```python
from build123d import *

# Parameters (mm, degrees)
SKETCH_1_R      = 3.05
SKETCH_1_R_2    = 2.25
EXTRUDE_1_DEPTH = 7
SKETCH_2_R      = 5
SKETCH_2_R_2    = 2.25
EXTRUDE_2_DEPTH = 2
EXTRUDE_START   = -2
SKETCH_3_R      = 5
SKETCH_3_R_2    = 2.25
EXTRUDE_3_DEPTH = 2
CHAMFER_1_SIZE  = 1.5


with BuildPart() as part:
    # Эскиз1 → Вытянуть-Тонкостенный1 (new body)
    with BuildSketch(Plane(origin=(0, 0, 0), x_dir=(1, 0, 0), z_dir=(0, 1, 0))):
        Circle(SKETCH_1_R)
        Circle(SKETCH_1_R_2, mode=Mode.SUBTRACT)
    extrude(amount=EXTRUDE_1_DEPTH)

    # Эскиз2 → Вытянуть-Тонкостенный2 (add)
    with BuildSketch(Plane(origin=(0, 0, 0), x_dir=(1, 0, 0), z_dir=(0, 1, 0))):
        Circle(SKETCH_2_R)
        Circle(SKETCH_2_R_2, mode=Mode.SUBTRACT)
    extrude(amount=EXTRUDE_2_DEPTH)

    # Эскиз3 → Вытянуть-Тонкостенный3 (add)
    with BuildSketch(Plane(origin=(0, 7, 0), x_dir=(1, 0, 0), z_dir=(0, 1, 0)).offset(EXTRUDE_START)):
        Circle(SKETCH_3_R)
        Circle(SKETCH_3_R_2, mode=Mode.SUBTRACT)
    extrude(amount=EXTRUDE_3_DEPTH)

    # Фаска1
    chamfer_1_edges = [part.edges().sort_by_distance(p)[0] for p in [
        (-3.05, 2, 0),
        (-3.05, 5, 0),
    ]]
    chamfer(chamfer_1_edges, length=CHAMFER_1_SIZE - 0.0001)  # a hair under: the kernel refuses the full size


solid = part.part
```
Model file for the job. Use its own axes, mm. Give positions to 0.01 mm unless a question says otherwise; leave off trailing zeros. Write each loop counter-clockwise with the first axis right and the second up, starting at its lowest first coordinate (ties: lowest second). Pieces come first, ordered by that corner, then holes. Notation, with made-up numbers: M 61,8.5 L 88,8.5 A13 cw 88,24.5 Z; hole C 21.5,-29.75 d7. An arc over 180 degrees is marked long. Use a Markdown table: item, result.
1) Pin check, flat tips, straight feed: pin 1 (3.5 mm diameter, centred on x = 0, z = 0, fed in from -Y); pin 2 (2 mm diameter, centred on x = 2.5, y = 1.5, fed in from +Z). Stop position of each tip, or through.
Responses:
| item | result |
|---|---|
| pin 1 | passes through |
| pin 2 | stops at z = 4.77 |
2) Pull direction Z, two halves, no side cores. Call faces 1 (the cylindrical face through (-1.08, 5.99, 4.88)), 2 (the cylindrical face through (-0.29, 3.45, -2.23)), 3 (the flat face through (2.2, 7, 1)): +Z half, -Z half, draft (parallel to the pull), parting line (faces both ways), or undercut.
Responses:
| item | result |
|---|---|
| face 1 | parting line |
| face 2 | undercut |
| face 3 | draft |
3) Drill centre lines: line 1 (Y direction, x = 2.5, z = 4); line 2 (X direction, y = 5.75, z = 0). Where is each one in solid material? Low to high. Write a range as from..to.
Responses:
| item | result |
|---|---|
| line 1 | y = 0..2, 5..7 |
| line 2 | x = -5..-2.25, 2.25..5 |
4) Cut at C-C (y = 0.5). List the corners of the cut face in (x, z), and give its area (3 significant figures).
Responses:
| item | result |
|---|---|
| outline | C 0,0 d10; hole C 0,0 d4.5 |
| area | 62.6 mm2 |
